from build123d import *

# Parameters (mm, degrees)
SKETCH1_R             = 2.925
SKETCH1_R_2           = 1.7499999999999998
MIDDLE_RING_DEPTH     = 0.8
SKETCH2_R             = 2.35
SKETCH2_R_2           = 1.7499999999999998
OUTER_BODY_DEPTH      = 7.35
SKETCH3_R             = 2.625
SKETCH3_R_2           = 1.7499999999999998
OUTER_RIM_DEPTH       = 0.5
SIDE_SLOTS_DEPTH      = 9.873204043636097
SIDE_SLOTS_DEPTH_BACK = 9.873204043636097
AXLE_START            = 15.95
AXLE_DEPTH            = 15.95
FILLET1_R             = 0.5
SKETCH7_R             = 2.925
AXLE_BASE_DEPTH       = 0.8


with BuildPart() as part:
    # Sketch1 → Middle Ring (new body)
    with BuildSketch(Plane(origin=(0, 0, 0), x_dir=(0, 0, -1), z_dir=(1, 0, 0))):
        Circle(SKETCH1_R)
        Circle(SKETCH1_R_2, mode=Mode.SUBTRACT)
    extrude(amount=MIDDLE_RING_DEPTH)

    # Sketch2 → Outer Body (add)
    with BuildSketch(Plane(origin=(0, 0, 0), x_dir=(0, 0, -1), z_dir=(1, 0, 0))):
        Circle(SKETCH2_R)
        Circle(SKETCH2_R_2, mode=Mode.SUBTRACT)
    extrude(amount=OUTER_BODY_DEPTH)

    # Sketch3 → Outer Rim (add)
    with BuildSketch(Plane(origin=(7.35, 0, 0), x_dir=(0, 0, -1), z_dir=(1, 0, 0))):
        Circle(SKETCH3_R)
        Circle(SKETCH3_R_2, mode=Mode.SUBTRACT)
    extrude(amount=OUTER_RIM_DEPTH)

    # Sketch5 → Side Slots (cut, two sides: drawn at the far end of the back side and taken through both)
    with BuildSketch(Plane(origin=(0, 0, 0), x_dir=(1, 0, 0), z_dir=(0, 1, 0)).offset(-SIDE_SLOTS_DEPTH_BACK)):
        with BuildLine():
            Line((10.949999999999998, -0.4999999999999999), (4.750000000000001, -0.4999999999999999))
            ThreePointArc((4.750000000000001, -0.4999999999999999), (4.250000000000006, 6e-17), (4.750000000000001, 0.4999999999999945))
            Line((4.750000000000001, 0.4999999999999945), (10.949999999999998, 0.4999999999999945))
            ThreePointArc((10.949999999999998, 0.4999999999999945), (11.449999999999998, 0), (10.949999999999998, -0.4999999999999999))
        make_face()
        with BuildLine():
            Line((-10.949999999999998, -0.4999999999999999), (-4.750000000000001, -0.4999999999999999))
            ThreePointArc((-4.750000000000001, -0.4999999999999999), (-4.250000000000006, 0), (-4.750000000000001, 0.4999999999999945))
            Line((-4.750000000000001, 0.4999999999999945), (-10.949999999999998, 0.4999999999999945))
            ThreePointArc((-10.949999999999998, 0.4999999999999945), (-11.449999999999998, -6e-17), (-10.949999999999998, -0.4999999999999999))
        make_face()
    extrude(amount=SIDE_SLOTS_DEPTH + SIDE_SLOTS_DEPTH_BACK, mode=Mode.SUBTRACT)

    # Sketch6 → Axle (add)
    with BuildSketch(Plane.ZY.offset(AXLE_START)):
        Polygon((-0.8999999999999999, -0.8999999999999999), (0.9000000000000001, -0.8999999999999999), (0.9000000000000001, 0.8999999999999999), (-0.8999999999999999, 0.9), align=None)
        with BuildLine():
            Line((-1.5008331019803216, -0.8999999999999999), (-0.8999999999999999, -0.8999999999999999))
            Line((-0.8999999999999999, -0.8999999999999999), (-0.8999999999999999, 0.8999999999999999))
            Line((-0.8999999999999999, 0.9), (-1.5008331019803216, 0.9))
            ThreePointArc((-1.500833101980337, 0.9000000000000439), (-1.7499999999999998, 2.1e-16), (-1.5008331019803371, -0.9000000000000435))
        make_face()
        with BuildLine():
            Line((-0.8999999999999999, 0.9), (0.9000000000000001, 0.9))
            Line((0.9000000000000001, 0.8999999999999999), (0.9000000000000001, 1.5008331019803842))
            ThreePointArc((0.8999999999999783, 1.5008331019803764), (-1.233e-14, 1.7499999999999998), (-0.8999999999999996, 1.5008331019803633))
            Line((-0.8999999999999999, 1.5008331019803633), (-0.8999999999999999, 0.8999999999999999))
        make_face()
        with BuildLine():
            Line((1.5008331019803591, -0.8999999999999999), (2.2248595461286844, -0.8999999999999999))
            ThreePointArc((2.22485954612869, -0.9000000000000218), (2.3558080259975402, -0.458441429896527), (2.4, -5.9e-16))
            ThreePointArc((2.4, 0), (2.3558080259975402, 0.45844142989652675), (2.2248595461286897, 0.9000000000000221))
            Line((2.224859546128683, 0.9), (1.5008331019803582, 0.9))
            ThreePointArc((1.5008331019803602, 0.900000000000005), (1.6865583192504239, 0.46692722748538085), (1.7499999999999998, 0))
            ThreePointArc((1.7499999999999998, -4.3e-16), (1.6865583192504237, -0.46692722748538135), (1.500833101980361, -0.900000000000004))
        make_face()
        with BuildLine():
            ThreePointArc((-2.4, 2.9e-16), (-2.3558080259975434, -0.45844142989651143), (-2.2248595461287017, -0.8999999999999924))
            Line((-2.224859546128704, -0.8999999999999999), (-1.5008331019803216, -0.8999999999999999))
            ThreePointArc((-1.5008331019803371, -0.9000000000000435), (-1.7499999999999998, 2.1e-16), (-1.500833101980337, 0.9000000000000439))
            Line((-1.5008331019803216, 0.9), (-2.224859546128704, 0.9))
            ThreePointArc((-2.2248595461287013, 0.899999999999994), (-2.355808025997543, 0.458441429896512), (-2.4, 2.9e-16))
        make_face()
        with BuildLine():
            ThreePointArc((-0.9000000000000059, -2.2248595461286964), (-0.4584414298964598, -2.355808025997553), (1.168e-13, -2.4))
            ThreePointArc((1.168e-13, -2.4), (0.45844142989653847, -2.355808025997538), (0.8999999999999359, -2.224859546128725))
            Line((0.9000000000000001, -2.224859546128744), (0.9000000000000001, -1.5008331019803836))
            ThreePointArc((0.899999999999978, -1.5008331019803764), (-1.276e-14, -1.7499999999999998), (-0.8999999999999986, -1.500833101980364))
            Line((-0.8999999999999999, -1.5008331019803647), (-0.8999999999999999, -2.2248595461286946))
        make_face()
        with BuildLine():
            ThreePointArc((-0.8999999999999996, 1.5008331019803633), (-1.233e-14, 1.7499999999999998), (0.8999999999999783, 1.5008331019803764))
            Line((0.9000000000000001, 1.5008331019803842), (0.9000000000000001, 2.2248595461287435))
            ThreePointArc((0.899999999999937, 2.2248595461287244), (0.4584414298965443, 2.355808025997537), (1.2698e-13, 2.4))
            ThreePointArc((1.2698e-13, 2.4), (-0.4584414298964561, 2.355808025997554), (-0.9000000000000058, 2.2248595461286964))
            Line((-0.8999999999999999, 2.2248595461286946), (-0.8999999999999999, 1.5008331019803633))
        make_face()
        with BuildLine():
            Line((0.9000000000000001, 0.8999999999999999), (0.9000000000000001, -0.8999999999999999))
            Line((0.9000000000000001, -0.8999999999999999), (1.5008331019803591, -0.8999999999999999))
            ThreePointArc((1.500833101980361, -0.900000000000004), (1.6865583192504237, -0.46692722748538135), (1.7499999999999998, -4.3e-16))
            ThreePointArc((1.7499999999999998, 0), (1.6865583192504239, 0.46692722748538085), (1.5008331019803602, 0.900000000000005))
            Line((1.5008331019803582, 0.9), (0.9000000000000001, 0.9))
        make_face()
        with BuildLine():
            ThreePointArc((-0.8999999999999986, -1.500833101980364), (-1.276e-14, -1.7499999999999998), (0.899999999999978, -1.5008331019803764))
            Line((0.9000000000000001, -1.5008331019803836), (0.9000000000000001, -0.8999999999999999))
            Line((0.9000000000000001, -0.8999999999999999), (-0.8999999999999999, -0.8999999999999999))
            Line((-0.8999999999999999, -0.8999999999999999), (-0.8999999999999999, -1.5008331019803647))
        make_face()
    extrude(amount=-AXLE_DEPTH)

    # Fillet1
    fillet1_edges = [part.edges().sort_by_distance(p)[0] for p in [
        (-15.95, -2.4, -2.377e-14),
        (-15.95, 7.1e-16, -2.4000000000000004),
        (-15.95, 2.4000000000000004, -2.279e-14),
        (-15.95, -1.1e-16, 2.4000000000000004),
    ]]
    fillet(fillet1_edges, radius=FILLET1_R)

    # Sketch7 → Axle Base (add)
    with BuildSketch(Plane.ZY):
        with Locations(Location((0, 0, 0), (0, 0, 180))):
            Circle(SKETCH7_R)
    extrude(amount=-AXLE_BASE_DEPTH)


solid = part.part
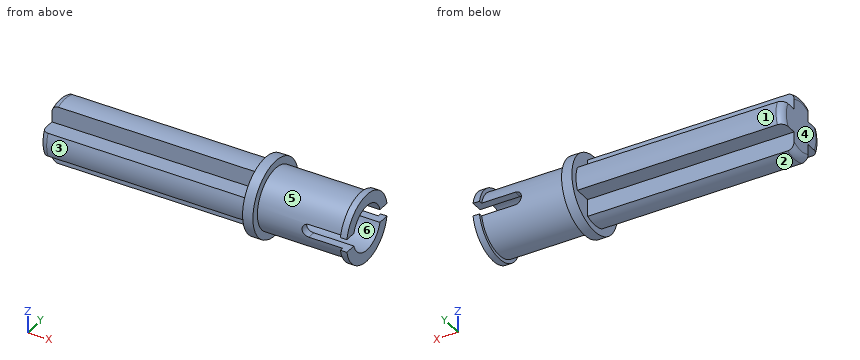
CAD build for the part. Positions are in the model's coordinates, mm. Face numbers are marked on the shaded views. A direction names the side the tool comes from. Give positions to 0.01 mm unless a question says otherwise; leave off trailing zeros. Order: outer loops, then holes, each group sorted by start corner. A loop starts at its lowest first (then second) coordinate and runs counter-clockwise, first axis right, second up. Notation, with made-up numbers: (-7, 29) -> (44, 29) arc R24 cw to (44, 41) -> close; hole circle Ø2 at (-34, 69.25). An arc over 180 degrees is marked (long way). Return JSON: item names as keys, results as strings.
Q1. Flat gauge pins, fed straight in: pin 1 (0.7 mm diameter, centred on x = -8.5, z = -1.5, fed in from +Y); pin 2 (1.1 mm diameter, centred on x = -5.5, z = -1.5, fed in from -Y); pin 3 (0.7 mm diameter, centred on x = 6.5, y = -2, fed in from -Z). Where does each tip first touch, or does it go through?
Working result:
{"pin 1": "y = 0.9", "pin 2": "y = -0.9", "pin 3": "z = -1.67"}
Q2. Saw through at D-D (z = 1.4). Write the cut outline in (x, y).
Working result:
{"outline": "(-15.95, -0.9) -> (0, -0.9) -> (0, -2.57) -> (0.8, -2.57) -> (0.8, -1.89) -> (7.35, -1.89) -> (7.35, -2.22) -> (7.85, -2.22) -> (7.85, -1.05) -> (0.8, -1.05) -> (0.8, 1.05) -> (7.85, 1.05) -> (7.85, 2.22) -> (7.35, 2.22) -> (7.35, 1.89) -> (0.8, 1.89) -> (0.8, 2.57) -> (0, 2.57) -> (0, 0.9) -> (-15.95, 0.9) -> close"}
Q3. Saw through at B-B (x = -11). Write the cut outline in (y, z), then the cut area to 3 significant figures.
Working result:
{"outline": "(-2.22, -0.9) -> (-0.9, -0.9) -> (-0.9, -2.22) arc R2.4 ccw to (0.9, -2.22) -> (0.9, -0.9) -> (2.22, -0.9) arc R2.4 ccw to (2.22, 0.9) -> (0.9, 0.9) -> (0.9, 2.22) arc R2.4 ccw to (-0.9, 2.22) -> (-0.9, 0.9) -> (-2.22, 0.9) arc R2.4 ccw to start", "area": "13.6 mm²"}
Q4. Which spindle directions (+Z, -Z, +X, -X, +Y, -Y) get a long thin tool onto all of the face, cutting with end or side? Do the marked faces 1, 2 and 3. Say none if no direction does.
Working result:
{"face 1": "-X, +Y", "face 2": "-Z, -X", "face 3": "-X, -Y"}
Q5. Mould opens along X. For the marked faces 4, 5 and 6 say: pulls with the +X half, pulls with the -X half, needs draft (parallel to the pull), parting line crosses it, or undercut.
Working result:
{"face 4": "pulls with the -X half", "face 5": "undercut", "face 6": "needs draft"}
Q6. Saw through at C-C (y = 0). Write the cut outline in (x, z) (3 decimals), then the cut area to 3 significant figures.
Working result:
{"outline": "(-15.95, -1.9) arc R0.5 ccw to (-15.45, -2.4) -> (0, -2.4) -> (0, -2.925) -> (0.8, -2.925) -> (0.8, -2.35) -> (7.35, -2.35) -> (7.35, -2.625) -> (7.85, -2.625) -> (7.85, -1.75) -> (0.8, -1.75) -> (0.8, 1.75) -> (7.85, 1.75) -> (7.85, 2.625) -> (7.35, 2.625) -> (7.35, 2.35) -> (0.8, 2.35) -> (0.8, 2.925) -> (0, 2.925) -> (0, 2.4) -> (-15.45, 2.4) arc R0.5 ccw to (-15.95, 1.9) -> close", "area": "89.9 mm²"}
Q7. Saw through at A-A (z = 0). Write the cut outline in (x, y) (3 decimals), then the cut area to 3 significant figures.
Working result:
{"outline": "(-15.95, -1.9) arc R0.5 ccw to (-15.45, -2.4) -> (0, -2.4) -> (0, -2.925) -> (0.8, -2.925) -> (0.8, -2.35) -> (4.25, -2.35) -> (4.25, -1.75) -> (0.8, -1.75) -> (0.8, 1.75) -> (4.25, 1.75) -> (4.25, 2.35) -> (0.8, 2.35) -> (0.8, 2.925) -> (0, 2.925) -> (0, 2.4) -> (-15.45, 2.4) arc R0.5 ccw to (-15.95, 1.9) -> close", "area": "85.3 mm²"}
Q8. Drill centre lines: line 1 (Z direction, x = 3.5, y = 0); line 2 (X direction, y = -1.8, z = -2.05). Where is each one in solid material? Low to high.
Working result:
{"line 1": "-2.35 to -1.75, 1.75 to 2.35", "line 2": "0 to 0.8"}
